Could you check a few things on this model? Use its own coordinates, in mm. Round coordinates to 2 decimals unless told otherwise and drop trailing zeros. Loops run counter-clockwise (first coordinate to the right, second up) from the corner with the lowest first, then second, coordinate; pieces in that order, holes last. Notation, with made-up numbers: (22, -5.75) -> (40, -5.75) arc R18 cw to (40, 22.25) -> close; hole circle Ø1 at (75, 34). An arc over 180 degrees is marked (long way). One line per item, written item: value.
```python
from build123d import *

# Parameters (mm, degrees)
F0_R = 2.7813
F3_R = 2.6055738226


with BuildPart() as f2:
    # F2: sweep along a path in F1
    with BuildLine(Plane.XY) as f2_path:
        Line((0, 0), (0, -19.05))
        ThreePointArc((0, -19.05), (-5.4271063194, -32.1521936806), (-18.5293, -37.5793))
        Line((-18.5293, -37.5793), (-24.8793, -37.5793))
    # F0 (on Front) → F2 (sweep)
    with BuildSketch(Plane.XZ):
        Circle(F0_R)
    sweep(path=f2_path.line)

    # F4: sweep along a path in F1
    with BuildLine(Plane.XY) as f4_path:
        Line((0, 0), (0, -19.05))
        ThreePointArc((0, -19.05), (-5.4271063194, -32.1521936806), (-18.5293, -37.5793))
        Line((-18.5293, -37.5793), (-24.8793, -37.5793))
    # F3 (on face) → F4 (sweep, cut)
    with BuildSketch(Plane(origin=(-24.8793, 0, 0), x_dir=(0, -1, 0), z_dir=(-1, 0, 0))):
        with Locations((37.5793, 0)):
            Circle(F3_R)
    sweep(path=f4_path.line, mode=Mode.SUBTRACT)


solid = f2.part
```
(1) Imagine slicing it at B-B on y = -7.5. Write out the boundary of the cut face in (x, z), then the cut area to 3 significant figures.
Results below:
outline: circle Ø5.56 at (0, 0); hole circle Ø5.21 at (0, 0)
area: 2.97 mm²
(2) Please list where these lines run through material, in increasing order: L1, parallel to Y at x = -21.25, z = 0; L2, parallel to X at y = -3.5, z = -0.1; L3, parallel to Z at x = 0, y = -7.5.
Results below:
L1: y = -40.36 to -40.18, -34.97 to -34.8
L2: x = -2.78 to -2.6, 2.6 to 2.78
L3: z = -2.78 to -2.61, 2.61 to 2.78
(3) We'd pull the mould along X, two halves only. Please class faces 1 (the face through (2.65, -9.66, 0.84)), 2 (the face through (2.485, -9.658, 0.783)), 3 (the face through (-21.749, -34.976, 0.115)): +X half, -X half, draft (parallel to the pull), parting line (faces both ways), or undercut.
Results below:
face 1: parting line
face 2: undercut
face 3: draft
(4) For pin 1 Ø2 at (x, z) = (-8, -1) entering from -Y; pin 2 Ø1 at (x, z) = (-13, 2) entering from +Y; pin 3 Ø10 at (x, y) = (-11, -28) entering from -Z, each with a flat end and sliding along its axis, tell me the tip position at first contact or that it passes through.
Results below:
pin 1: stops at y = -38
pin 2: stops at y = -34.22
pin 3: stops at z = -2.09
(5) Imagine slicing it at C-C on x = -22.25. Write out the boundary of the cut face in (y, z).
Results below:
outline: circle Ø5.56 at (-37.58, 0); hole circle Ø5.21 at (-37.58, 0)
(6) Imagine slicing it at A-A on z = 0. Write out the boundary of the cut face in (x, y).
Results below:
outline: (-24.88, -40.36) -> (-18.53, -40.36) arc R21.31 ccw to (2.78, -19.05) -> (2.78, 0) -> (2.61, 0) -> (2.61, -19.05) arc R21.13 cw to (-18.53, -40.18) -> (-24.88, -40.18) -> close; (-24.88, -34.97) -> (-18.53, -34.97) arc R15.92 ccw to (-2.61, -19.05) -> (-2.61, 0) -> (-2.78, 0) -> (-2.78, -19.05) arc R15.75 cw to (-18.53, -34.8) -> (-24.88, -34.8) -> close
